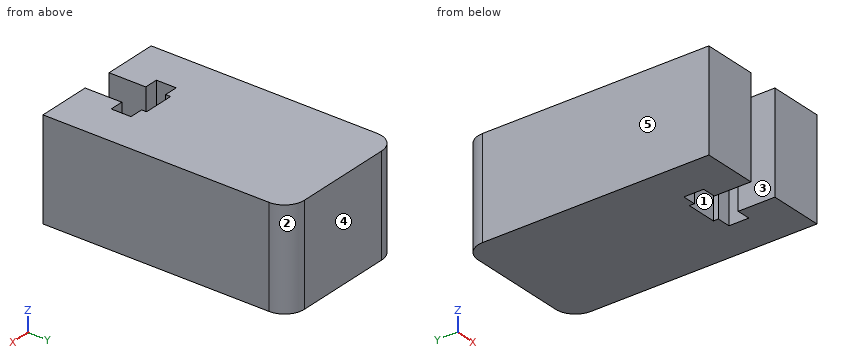
from build123d import *

# Parameters (mm, degrees)
DODANIE_WYCI_GNI_CIE1_DEPTH = 10
WYTNIJ_WYCI_GNI_CIE1_DEPTH  = 10


with BuildPart() as part:
    # Szkic1 → Dodanie-wyciągnięcie1 (new body)
    with BuildSketch(Plane.XY):
        with BuildLine():
            Line((-46.47600649, 4), (-60.47600649, 4))
            Line((-60.47600649, 4), (-60.47600649, 26.8))
            ThreePointArc((-60.47600649, 26.8), (-59.890220053, 28.214213562), (-58.47600649, 28.8))
            Line((-58.47600649, 28.8), (-48.47600649, 28.8))
            ThreePointArc((-48.47600649, 28.8), (-47.061792928, 28.214213562), (-46.47600649, 26.8))
            Line((-46.47600649, 26.8), (-46.47600649, 4))
        make_face()
    extrude(amount=DODANIE_WYCI_GNI_CIE1_DEPTH)

    # Szkic3 → Wytnij-wyciągnięcie1 (cut)
    with BuildSketch(Plane.XY.offset(10)):
        Polygon((-51.92600649, 4), (-55.02600649, 4), (-55.02600649, 7.7), (-56.40100649, 7.7), (-56.40100649, 9.7), (-55.02600649, 9.7), (-55.02600649, 10.2), (-51.92600649, 10.2), (-51.92600649, 9.7), (-50.55100649, 9.7), (-50.55100649, 7.7), (-51.92600649, 7.7), align=None)
    extrude(amount=-WYTNIJ_WYCI_GNI_CIE1_DEPTH, mode=Mode.SUBTRACT)


solid = part.part
Input: part model. Units: mm. Frame: model coordinates. Face numbers are marked on the shaded views. A direction names the side the tool comes from. Give positions to 0.01 mm unless a question says otherwise; leave off trailing zeros. Order: outer loops, then holes, each group sorted by start corner. A loop starts at its lowest first (then second) coordinate and runs counter-clockwise, first axis right, second up. Notation, with made-up numbers: (58, 62) - (67, 62) arc R13 ccw to (67, 80) - close; hole circle Ø6 at (55.5, 56.5). An arc over 180 degrees is marked (long way). Answer as a JSON object with one key per item and string values. Group by question number.
Q1. Cut plane C-C, the plane x = -53. Output: boundary loops of the cut face in (y, z).
Q2. Mould query, pull axis X, two halves, no side actions, for the marked faces 3, 4 and 5. Classes: pulls with the +X half, pulls with the -X half, needs draft (parallel to the pull), parting line crosses it, or undercut.
Q3. Cut plane B-B, the plane z = 2.5. Output: boundary loops of the cut face in (x, y), then the cut area to 3 significant figures.
Q4. Set-up query: the marked faces 1 and 2. Return all of +Z, -Z, +X, -X, +Y, -Y with unobstructed straight access to the full face (end or side cutting, diameter ignored); none if empty.
Q5. Cut plane A-A, the plane y = 8.25. Output: boundary loops of the cut face in (x, z), then the cut area to 3 significant figures.
Q6. Line query: probe 1 along Y at (x, z) = (-51, 5); probe 2 along X at (y, z) = (10, 0.75); probe 3 along X at (y, z) = (9.5, 5). Output: solid intervals per line, ascending.
Results:
{
 "1": {"outline": "(10.2, 0) - (28.8, 0) - (28.8, 10) - (10.2, 10) - close"},
 "2": {"face 3": "undercut", "face 4": "needs draft", "face 5": "pulls with the -X half"},
 "3": {"outline": "(-60.48, 4) - (-55.03, 4) - (-55.03, 7.7) - (-56.4, 7.7) - (-56.4, 9.7) - (-55.03, 9.7) - (-55.03, 10.2) - (-51.93, 10.2) - (-51.93, 9.7) - (-50.55, 9.7) - (-50.55, 7.7) - (-51.93, 7.7) - (-51.93, 4) - (-46.48, 4) - (-46.48, 26.8) arc R2 ccw to (-48.48, 28.8) - (-58.48, 28.8) arc R2 ccw to (-60.48, 26.8) - close", "area": "321 mm^2"},
 "4": {"face 1": "+Z, -Z, -Y", "face 2": "+Z, -Z, +X, +Y"},
 "5": {"outline": "(-60.48, 0) - (-56.4, 0) - (-56.4, 10) - (-60.48, 10) - close; (-50.55, 0) - (-46.48, 0) - (-46.48, 10) - (-50.55, 10) - close", "area": "81.5 mm^2"},
 "6": {"probe 1": "4 to 7.7, 9.7 to 28.8", "probe 2": "-60.48 to -55.03, -51.93 to -46.48", "probe 3": "-60.48 to -56.4, -50.55 to -46.48"}
}
